Geometry check sheet. Reference: the model listing, model coordinates, mm. A direction names the side the tool comes from. Give positions to 0.01 mm unless a question says otherwise; leave off trailing zeros. Write each loop counter-clockwise with the first axis right and the second up, starting at its lowest first coordinate (ties: lowest second). Pieces come first, ordered by that corner, then holes. Notation, with made-up numbers: M -14,76.25 L 33,76.25 A11 ccw 33,92.25 Z; hole C 18.25,66 d6. An arc over 180 degrees is marked long. Write each question's results on one line, items separated by ' | '.
```python
from build123d import *

# Parameters (mm, degrees)
F3_DEPTH     = 10.0076
F4_DEPTH     = 40.005
F6_START     = -19.9898
F6_DEPTH     = 10.0076
F7_DEPTH     = 10.0076
F9_START     = 20.2438
F2_R         = 3.2004
F9_DEPTH     = 9.4996
F10_DEPTH    = 10.2616
F11_START    = 20.0152
F11_DEPTH    = 9.9822
F12_START    = -19.7612
F12_DEPTH    = 11.6078
F13_DEPTH    = 9.7536
F14_T1_DEPTH = 13.1863686745
F15_T1_DEPTH = 65.405
F16_R        = 2.54


# Not quite as in the source:
# - a fillet or chamfer that OpenCascade refuses, or shapes differently, is made with other operations: its cross-section is extruded or revolved along the edge and cut away or added


with BuildPart() as f3:
    # F0 (on Front) → F3 (new body)
    with BuildSketch(Plane.XZ):
        with BuildLine():
            ThreePointArc((-4.8989745866, 2.54), (-2.7591462448, 0.6727514434), (0, 0))
            ThreePointArc((0, 0), (3.8726462994, 1.4188735822), (5.9119830007, 5.0038))
            ThreePointArc((5.9119830007, 5.0038), (5.9737602169, 5.4973887019), (5.9944, 5.9944))
            ThreePointArc((5.9944, 5.9944), (-1.8119627615, 11.7083848014), (-4.8989745866, 2.54))
        make_face()
        with BuildLine():
            ThreePointArc((-0.3048, 3.0127385839), (0, 8.9916), (0.3048, 3.0127385839))
            Line((0.3048, 3.0127385839), (0.3048, 2.808547348))
            ThreePointArc((0.3048, 2.808547348), (0, 2.794), (-0.3048, 2.808547348))
            Line((-0.3048, 2.808547348), (-0.3048, 3.0127385839))
        make_face(mode=Mode.SUBTRACT)
        with BuildLine():
            Line((-12.5189745866, 0), (0, 0))
            ThreePointArc((0, 0), (-2.7591462448, 0.6727514434), (-4.8989745866, 2.54))
            Line((-4.8989745866, 2.54), (-12.5189745866, 2.54))
            Line((-12.5189745866, 2.54), (-12.5189745866, 0))
        make_face()
    extrude(amount=-F3_DEPTH)

    # F0 (on Front) → F4 (join)
    with BuildSketch(Plane.XZ):
        with BuildLine():
            Line((0.3048, 2.808547348), (0.3048, 3.0127385839))
            ThreePointArc((0.3048, 3.0127385839), (0, 8.9916), (-0.3048, 3.0127385839))
            Line((-0.3048, 3.0127385839), (-0.3048, 2.808547348))
            ThreePointArc((-0.3048, 2.808547348), (0, 2.794), (0.3048, 2.808547348))
        make_face()
    extrude(amount=-F4_DEPTH)

    # F0 (on Front) → F6 (join)
    with BuildSketch(Plane.XZ.offset(F6_START)):
        with BuildLine():
            ThreePointArc((-4.8989745866, 2.54), (-2.7591462448, 0.6727514434), (0, 0))
            ThreePointArc((0, 0), (3.8726462994, 1.4188735822), (5.9119830007, 5.0038))
            ThreePointArc((5.9119830007, 5.0038), (5.9737602169, 5.4973887019), (5.9944, 5.9944))
            ThreePointArc((5.9944, 5.9944), (-1.8119627615, 11.7083848014), (-4.8989745866, 2.54))
        make_face()
        with BuildLine():
            ThreePointArc((-0.3048, 3.0127385839), (0, 8.9916), (0.3048, 3.0127385839))
            Line((0.3048, 3.0127385839), (0.3048, 2.808547348))
            ThreePointArc((0.3048, 2.808547348), (0, 2.794), (-0.3048, 2.808547348))
            Line((-0.3048, 2.808547348), (-0.3048, 3.0127385839))
        make_face(mode=Mode.SUBTRACT)
        with BuildLine():
            Line((-12.5189745866, 0), (0, 0))
            ThreePointArc((0, 0), (-2.7591462448, 0.6727514434), (-4.8989745866, 2.54))
            Line((-4.8989745866, 2.54), (-12.5189745866, 2.54))
            Line((-12.5189745866, 2.54), (-12.5189745866, 0))
        make_face()
    extrude(amount=-F6_DEPTH)

    # F2 (on offset) → F7 (join)
    with BuildSketch(Plane.XZ.offset(-40.005)):
        with BuildLine():
            ThreePointArc((-1.5118372742, 0.1937811178), (-3.4133287183, 1.0667211934), (-4.8989745866, 2.54))
            Line((-4.8989745866, 2.54), (-12.5189745866, 2.54))
            Line((-12.5189745866, 2.54), (-12.5189745866, 0))
            Line((-12.5189745866, 0), (-1.5366753453, 0))
            ThreePointArc((-1.5366753453, 0), (-1.4389921182, 0.0859617436), (-1.5118372742, 0.1937811178))
        make_face()
    extrude(amount=F7_DEPTH)

    # F2 (on offset) → F9 (join)
    with BuildSketch(Plane.XZ.offset(-40.005).offset(F9_START)):
        with BuildLine():
            Line((0, 0.3048), (0, 0))
            ThreePointArc((0, 0), (3.8726462994, 1.4188735822), (5.9119830007, 5.0038))
            Line((5.9119830007, 5.0038), (5.6027011164, 5.0038))
            ThreePointArc((5.6027011164, 5.0038), (-3.6561886166, 10.353738592), (0, 0.3048))
        make_face()
        with Locations((0, 5.9944)):
            Circle(F2_R, mode=Mode.SUBTRACT)
        with BuildLine():
            ThreePointArc((5.9119830007, 5.0038), (3.8726462994, 1.4188735822), (0, 0))
            Line((0, 0), (19.9898, 0))
            Line((19.9898, 0), (19.9898, 5.0038))
            Line((19.9898, 5.0038), (5.9119830007, 5.0038))
        make_face()
    extrude(amount=F9_DEPTH)

    # F0 (on Front) → F10 (join)
    with BuildSketch(Plane.XZ):
        with BuildLine():
            ThreePointArc((6.2722573002, 5.0038), (4.8747199854, 1.9250505355), (2.0951536077, 0))
            Line((2.0951536077, 0), (19.9898, 0))
            Line((19.9898, 0), (19.9898, 5.0038))
            Line((19.9898, 5.0038), (6.2722573002, 5.0038))
        make_face()
    extrude(amount=-F10_DEPTH)

    # F2 (on offset) → F11 (join)
    with BuildSketch(Plane.XZ.offset(-40.005).offset(F11_START)):
        with BuildLine():
            ThreePointArc((-1.5118372742, 0.1937811178), (-3.4133287183, 1.0667211934), (-4.8989745866, 2.54))
            Line((-4.8989745866, 2.54), (-12.5189745866, 2.54))
            Line((-12.5189745866, 2.54), (-12.5189745866, 0))
            Line((-12.5189745866, 0), (-1.5366753453, 0))
            ThreePointArc((-1.5366753453, 0), (-1.4389921182, 0.0859617436), (-1.5118372742, 0.1937811178))
        make_face()
    extrude(amount=F11_DEPTH)

    # F0 (on Front) → F12 (join)
    with BuildSketch(Plane.XZ.offset(F12_START)):
        with BuildLine():
            ThreePointArc((6.2722573002, 5.0038), (4.8747199854, 1.9250505355), (2.0951536077, 0))
            Line((2.0951536077, 0), (19.9898, 0))
            Line((19.9898, 0), (19.9898, 5.0038))
            Line((19.9898, 5.0038), (6.2722573002, 5.0038))
        make_face()
    extrude(amount=-F12_DEPTH)

    # F2 (on offset) → F13 (join)
    with BuildSketch(Plane.XZ.offset(-40.005)):
        with BuildLine():
            ThreePointArc((5.9119830007, 5.0038), (3.8726462994, 1.4188735822), (0, 0))
            Line((0, 0), (19.9898, 0))
            Line((19.9898, 0), (19.9898, 5.0038))
            Line((19.9898, 5.0038), (5.9119830007, 5.0038))
        make_face()
        with BuildLine():
            Line((0, 0.3048), (0, 0))
            ThreePointArc((0, 0), (3.8726462994, 1.4188735822), (5.9119830007, 5.0038))
            Line((5.9119830007, 5.0038), (5.6027011164, 5.0038))
            ThreePointArc((5.6027011164, 5.0038), (-3.6561886166, 10.353738592), (0, 0.3048))
        make_face()
        with Locations((0, 5.9944)):
            Circle(F2_R, mode=Mode.SUBTRACT)
    extrude(amount=F13_DEPTH)

    # F14: fillet of radius 0.254 on 1 edges, made by hand

    # F14_s2 → F14_t1 (cut)
    with BuildSketch(Plane.XZ.offset(-10.2616)):
        with BuildLine():
            ThreePointArc((3.1394818053, 0.4747846154), (3.0195052872, 0.1890511444), (3.2650610775, 0))
            Line((3.2650610775, 0), (2.0951536077, 0))
            ThreePointArc((2.0951536077, 0), (2.628061469, 0.2137605098), (3.1394818053, 0.4747846154))
        make_face()
    extrude(amount=F14_T1_DEPTH, mode=Mode.SUBTRACT)

    # F15: fillet of radius 5.08 on 1 edges, made by hand

    # F15_s2 → F15_t1 (cut)
    with BuildSketch(Plane.XZ.offset(-52.705)):
        with BuildLine():
            ThreePointArc((19.9898, -0.0762), (18.5019024484, 3.5159024484), (14.9098, 5.0038))
            Line((14.9098, 5.0038), (19.9898, 5.0038))
            Line((19.9898, 5.0038), (19.9898, -0.0762))
        make_face()
    extrude(amount=F15_T1_DEPTH, mode=Mode.SUBTRACT)

    # F16
    f16_edges = [f3.edges().sort_by_distance(p)[0] for p in [
        (10.256251, 40.005, 5.0038),
        (10.591029, 0, 5.0038),
        (18.47486, 40.005, 3.542743),
        (18.47486, 0, 3.542743),
    ]]
    fillet(f16_edges, radius=F16_R)


solid = f3.part
```
Q1. Section check B-B (y = 21.5). Enter the section's corners in (x, z).
Answer key:
outline: M -12.52,0 L 0,0 A5.99 ccw long -4.9,2.54 L -12.52,2.54 Z; M 2.1,0 L 19.99,0 A5.08 ccw 14.91,5 L 6.27,5 A6.35 cw Z
Q2. Material ranges on probe 1 along X at (y, z) = (35, 6.25); probe 2 along Y at (x, z) = (-4, 2.25) (3 decimals); probe 3 along Y at (x, z) = (3.5, 1) (3 decimals), recorded low to high. Write a range as [from, to].
Answer key:
probe 1: x = [-5.68, -3.19], [-2.99, 2.99], [3.19, 5.68] | probe 2: y = [0, 10.008], [10.262, 19.761], [19.99, 29.997], [30.251, 40.005] | probe 3: y = [10.262, 19.761], [30.251, 40.005]
Q3. Section check C-C (z = 7.5). State how many separate pieces and enclosed holes the cut face has, then the cut area to 3 significant figures.
Answer key:
separate pieces: 5 | enclosed holes: 0 | area: 438 mm2
Q4. Section check A-A (y = 34). Enter the section's corners in (x, z), then the cut area to 3 significant figures.
Answer key:
outline: M -12.52,0 L -1.54,0 A0.1 ccw -1.51,0.19 A5.99 cw -4.9,2.54 L -12.52,2.54 Z; M 0,0 L 19.99,0 A5.08 ccw 14.91,5 L 5.6,5 A5.69 ccw long 0,0.3 Z; hole M -0.3,2.81 L -0.3,3.01 A3 cw long 0.3,3.01 L 0.3,2.81 A3.2 ccw long Z | area: 196 mm2
Q5. Section check D-D (x = 4). Enter the section's corners in (y, z) (3 decimals), then the cut area to 3 significant figures.
Answer key:
outline: M 0,0 L 40.005,0 L 40.005,10.041 L 30.251,10.041 L 30.251,1.063 L 19.761,1.063 L 19.761,10.041 L 10.262,10.041 L 10.262,1.063 L 0,1.063 Z; M 0,1.53 L 10.008,1.53 L 10.008,10.459 L 0,10.459 Z; M 19.99,1.53 L 29.997,1.53 L 29.997,10.459 L 19.99,10.459 Z | area: 394 mm2
Q6. Release check for a two-part mould opening along Z. For faces 1 (the face through (18.514, 20.247, 3.504)), 2 (the face through (4.905, 24.933, 1.962)), 3 (the face through (-4.82, 35.2, 9.02)), 4 (the face through (-8, 40.005, 1)) record: released by +Z, released by -Z, zero draft, split by the parting line, or undercut.
Answer key:
face 1: released by +Z | face 2: undercut | face 3: undercut | face 4: zero draft
Q7. Depth check by flat-ended pin: P1, Ø7.5, axis at x = 11.5, y = 19, coming from the +Z side; P2, Ø3, axis at y = 4.5, z = 10, coming from the -X side. Enter the tip coordinate at first touch or a pass-through.
Answer key:
P1: stops at z = 5 | P2: stops at x = -5.45
Q8. Access from +Z, -Z, +X, -X, +Y, -Y to the whole of each face (thin tool, end or side, straight path). Record for faces 5 (the face through (0.13, 34.93, 8.99)), 6 (the face through (10, 20, 0)), 7 (the face through (-3.5, 15.08, 10.48)).
Answer key:
face 5: +Y | face 6: -Z, +X, -X, +Y, -Y | face 7: none
